from build123d import *

# Parameters (mm, degrees)
F1_DEPTH = 3


with BuildPart() as f1:
    # F0 (on Front) → F1 (new body)
    with BuildSketch(Plane.XZ):
        with BuildLine():
            Line((-14.5, 31.302889), (-17.5, 31.302889))
            ThreePointArc((-17.5, 31.302889), (-20.328427, 30.131316), (-21.5, 27.302889))
            Line((-21.5, 27.302889), (-21.5, 15.302889))
            ThreePointArc((-21.5, 15.302889), (-20.328427, 12.474462), (-17.5, 11.302889))
            Line((-17.5, 11.302889), (-3, 11.302889))
            Line((-3, 11.302889), (-3, 21.302889))
            Line((-3, 21.302889), (0, 21.302889))
            Line((0, 21.302889), (0, 11.302889))
            Line((0, 11.302889), (14.5, 11.302889))
            ThreePointArc((14.5, 11.302889), (17.328427, 12.474462), (18.5, 15.302889))
            Line((18.5, 15.302889), (18.5, 27.302889))
            ThreePointArc((18.5, 27.302889), (17.328427, 30.131316), (14.5, 31.302889))
            Line((14.5, 31.302889), (11.5, 31.302889))
            Line((11.5, 31.302889), (11.5, 21.302889))
            Line((11.5, 21.302889), (8.5, 21.302889))
            Line((8.5, 21.302889), (8.5, 31.302889))
            Line((8.5, 31.302889), (-11.5, 31.302889))
            Line((-11.5, 31.302889), (-11.5, 21.302889))
            Line((-11.5, 21.302889), (-14.5, 21.302889))
            Line((-14.5, 21.302889), (-14.5, 31.302889))
        make_face()
    extrude(amount=F1_DEPTH)


solid = f1.part
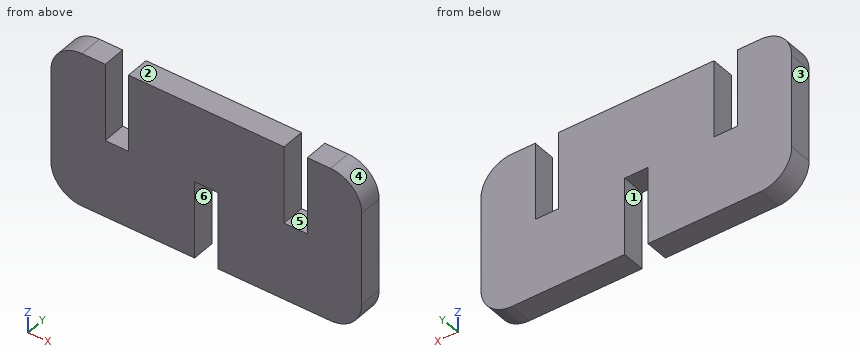
CAD build for the part. Positions are in the model's coordinates, mm. Face numbers are marked on the shaded views. A direction names the side the tool comes from. Give positions to 0.01 mm unless a question says otherwise; leave off trailing zeros. Loops run counter-clockwise (first coordinate to the right, second up) from the corner with the lowest first, then second, coordinate; pieces in that order, holes last. Notation, with made-up numbers: M -30.75,-22.5 L 16.25,-22.5 A29 cw 16.25,16.5 Z; hole C -3.5,44 d7. An arc over 180 degrees is marked long. Answer in a Markdown table with one row per item. Add a question column.
Item 1: Probe probe 1 along X at (y, z) = (-1.95, 26.5); probe 2 along X at (y, z) = (-1.3, 15.5); probe 3 along X at (y, z) = (-2.45, 28.5). List the from-to ranges inside material, lowest first.
Item 2: Band-saw the part on D-D on x = -14. Give the cut face in (y, z).
Item 3: Mould opens along X. For the marked faces 1, 2 and 3 say: +X half, -X half, draft (parallel to the pull), parting line (faces both ways), or undercut.
Item 4: Band-saw the part on B-B on y = -1.8. Give the cut face in (x, z), then the cut area to 3 significant figures.
Item 5: Tool access for the marked faces 4, 5 and 6: list every direction of +Z, -Z, +X, -X, +Y, -Y with a clear straight run to the whole face (end or side of a thin tool).
Item 6: Band-saw the part on C-C on z = 29.5. Give the cut face in (x, y), then the cut area to 3 significant figures.
Item 7: Drop flat-ended pins along their axis: P1, Ø12, axis at x = 11, z = 29, coming from the +Y side; P2, Ø0.9, axis at x = -1.5, y = -1.5, coming from the -Z side; P3, Ø1.5, axis at x = -12.5, y = -1.5, coming from the +Z side. Give the stop position or say it passes through.
Item 8: Band-saw the part on A-A on z = 13.25. Give the cut face in (x, y).
Reply:
| question | item | result |
|---|---|---|
| 1 | probe 1 | x = -21.5 to -14.5, -11.5 to 8.5, 11.5 to 18.5 |
| 1 | probe 2 | x = -21.5 to -3, 0 to 18.5 |
| 1 | probe 3 | x = -21.32 to -14.5, -11.5 to 8.5, 11.5 to 18.32 |
| 2 | outline | M -3,11.3 L 0,11.3 L 0,21.3 L -3,21.3 Z |
| 3 | face 1 | undercut |
| 3 | face 2 | draft |
| 3 | face 3 | -X half |
| 4 | outline | M -21.5,15.3 A4 ccw -17.5,11.3 L -3,11.3 L -3,21.3 L 0,21.3 L 0,11.3 L 14.5,11.3 A4 ccw 18.5,15.3 L 18.5,27.3 A4 ccw 14.5,31.3 L 11.5,31.3 L 11.5,21.3 L 8.5,21.3 L 8.5,31.3 L -11.5,31.3 L -11.5,21.3 L -14.5,21.3 L -14.5,31.3 L -17.5,31.3 A4 ccw -21.5,27.3 Z |
| 4 | area | 696 mm^2 |
| 5 | face 4 | +Z, +X, +Y, -Y |
| 5 | face 5 | +Z, +Y, -Y |
| 5 | face 6 | -Z, +Y, -Y |
| 6 | outline | M -20.84,-3 L -14.5,-3 L -14.5,0 L -20.84,0 Z; M -11.5,-3 L 8.5,-3 L 8.5,0 L -11.5,0 Z; M 11.5,-3 L 17.84,-3 L 17.84,0 L 11.5,0 Z |
| 6 | area | 98.1 mm^2 |
| 7 | P1 | stops at y = 0 |
| 7 | P2 | stops at z = 21.3 |
| 7 | P3 | stops at z = 21.3 |
| 8 | outline | M -20.93,-3 L -3,-3 L -3,0 L -20.93,0 Z; M 0,-3 L 17.93,-3 L 17.93,0 L 0,0 Z |
